Source: CAD feature listing. Evaluate the final solid. Frame: model axes, mm. A direction names the side the tool comes from. Round coordinates to 2 decimals unless told otherwise and drop trailing zeros. Write each loop counter-clockwise with the first axis right and the second up, starting at its lowest first coordinate (ties: lowest second). Pieces come first, ordered by that corner, then holes. Notation, with made-up numbers: M 32.5,66.25 L 74.5,66.25 A10 ccw 74.5,85.25 Z; hole C 8.25,67.5 d1. An arc over 180 degrees is marked long. Answer in a Markdown table with one row per item.
from build123d import *

# Parameters (mm, degrees)
SKETCH3_R          = 14.674629281
CUT_EXTRUDE1_DEPTH = 6.35
SKETCH4_W          = 6.858
SKETCH4_H          = 15.764878236
CUT_EXTRUDE2_DEPTH = 50.8
SKETCH7_W          = 3.175
SKETCH7_H          = 17.78
FINGERGRIP_DEPTH   = 1.651
GRIPS_START        = -20.955
GRIPS_DEPTH        = 17.78


# Read off the part's stored shape, not the designer's step: grips
with BuildPart() as part:
    # Sketch1 → Revolve3 (revolve)
    with BuildSketch(Plane(origin=(0, 0, 0), x_dir=(0, 0, -1), z_dir=(1, 0, 0)), mode=Mode.PRIVATE) as revolve3_sk:
        Polygon((54.61, 12.700000001), (54.61, 10.16), (41.91, 10.16), (22.86, 13.384649532), (0, 13.384649532), (0, 16.51), (22.86, 16.51), (41.91, 12.700000001), align=None)
    revolve(revolve3_sk.sketch.rotate(Axis((0, 0, 0), (0, 0, -1)), 90), axis=Axis((0, 0, 0), (0, 0, -1)))

    # Sketch3 → Cut-Extrude1 (cut)
    with BuildSketch(Plane.XY):
        Circle(SKETCH3_R)
    extrude(amount=-CUT_EXTRUDE1_DEPTH, mode=Mode.SUBTRACT)

    # Sketch4 → Cut-Extrude2 (cut, symmetric)
    with BuildSketch(Plane(origin=(0, 0, 0), x_dir=(0, 0, -1), z_dir=(1, 0, 0))):
        with Locations((47.117, 7.882439118)):
            Rectangle(SKETCH4_W, SKETCH4_H)
    extrude(amount=CUT_EXTRUDE2_DEPTH, both=True, mode=Mode.SUBTRACT)

    # Sketch7 → fingerGrip (add)
    with BuildSketch(Plane(origin=(0, 15.875, 0), x_dir=(-1, 0, 0), z_dir=(0, 1, 0))):
        with Locations((0, -12.065)):
            Rectangle(SKETCH7_W, SKETCH7_H)
    extrude(amount=FINGERGRIP_DEPTH)

    # grips outline → grips (add)
    with BuildSketch(Plane.XY.offset(GRIPS_START)):
        with BuildLine():
            Line((1.5875, -17.526), (1.5875, -16.433500654))
            ThreePointArc((1.5875, -16.433500654), (0, -16.51), (-1.5875, -16.433500654))
            Line((-1.5875, -16.433500654), (-1.5875, -17.526))
            Line((-1.5875, -17.526), (1.5875, -17.526))
        make_face()
        with BuildLine():
            ThreePointArc((15.02557904, -6.841934999), (14.298079416, -8.255), (13.43807904, -9.591565656))
            Line((13.43807904, -9.591565656), (14.384211227, -10.137815329))
            Line((14.384211227, -10.137815329), (15.971711227, -7.388184671))
            Line((15.971711227, -7.388184671), (15.02557904, -6.841934999))
        make_face()
        with BuildLine():
            Line((-14.384211227, -10.137815329), (-13.43807904, -9.591565656))
            ThreePointArc((-13.43807904, -9.591565656), (-14.298079416, -8.255), (-15.02557904, -6.841934999))
            Line((-15.02557904, -6.841934999), (-15.971711227, -7.388184671))
            Line((-15.971711227, -7.388184671), (-14.384211227, -10.137815329))
        make_face()
        with BuildLine():
            Line((-15.971711227, 7.388184671), (-15.02557904, 6.841934999))
            ThreePointArc((-15.02557904, 6.841934999), (-14.298079416, 8.255), (-13.43807904, 9.591565656))
            Line((-13.43807904, 9.591565656), (-14.384211227, 10.137815329))
            Line((-14.384211227, 10.137815329), (-15.971711227, 7.388184671))
        make_face()
        with BuildLine():
            ThreePointArc((13.43807904, 9.591565656), (14.298079416, 8.255), (15.02557904, 6.841934999))
            Line((15.02557904, 6.841934999), (15.971711227, 7.388184671))
            Line((15.971711227, 7.388184671), (14.384211227, 10.137815329))
            Line((14.384211227, 10.137815329), (13.43807904, 9.591565656))
        make_face()
    extrude(amount=GRIPS_DEPTH)


solid = part.part
Q1. Contact query for flat-ended pins moving along their axis: pin 1 Ø6 at (y, z) = (-9, -33) entering from -X; pin 2 Ø10 at (x, y) = (-9.5, -7) entering from +Z; pin 3 Ø0.9 at (y, z) = (17, -16.5) entering from -X; pin 4 Ø3 at (y, z) = (11, -9) entering from -X. Output: stop coordinate, or through.
Solutions:
| item | result |
|---|---|
| pin 1 | stops at x = -13.33 |
| pin 2 | stops at z = 0 |
| pin 3 | stops at x = -1.59 |
| pin 4 | stops at x = -14.75 |
Q2. Material intervals for probe 1 along Y at (x, z) = (0, -13); probe 2 along Y at (x, z) = (0, -3); probe 3 along X at (y, z) = (7, -42), sorted ascending.
Solutions:
| item | result |
|---|---|
| probe 1 | y = -17.53 to -13.38, 13.38 to 17.53 |
| probe 2 | y = -16.51 to -14.67, 14.67 to 16.51 |
| probe 3 | x = -10.6 to -7.36, 7.36 to 10.6 |
Q3. Access query for faces 4 (the flat face through (14.7, 8.5, -3.175)), 5 (the flat face through (0, 11, -43.688)), 6 (the flat face through (-1.588, 17, -12)), 7 (the flat face through (1.588, -17, -12)). Directions: +Z, -Z, +X, -X, +Y, -Y. A direction counts if a zero-diameter tool reaches every point of the face in a straight line with its end or side. Return the directions, or none.
Solutions:
| item | result |
|---|---|
| face 4 | +Z, +X, +Y |
| face 5 | +X, -X, +Y |
| face 6 | +Z, -Z, -X, +Y |
| face 7 | +Z, -Z, +X, -Y |
Q4. Section B-B (z = -15.5). Return loops of the section in (x, y).
Solutions:
| item | result |
|---|---|
| outline | M -15.97,-7.39 L -14.38,-10.14 L -13.44,-9.59 A16.51 ccw -1.59,-16.43 L -1.59,-17.53 L 1.59,-17.53 L 1.59,-16.43 A16.51 ccw 13.44,-9.59 L 14.38,-10.14 L 15.97,-7.39 L 15.03,-6.84 A16.51 ccw 15.03,6.84 L 15.97,7.39 L 14.38,10.14 L 13.44,9.59 A16.51 ccw 1.59,16.43 L 1.59,17.53 L -1.59,17.53 L -1.59,16.43 A16.51 ccw -13.44,9.59 L -14.38,10.14 L -15.97,7.39 L -15.03,6.84 A16.51 ccw -15.03,-6.84 Z; hole C 0,0 d26.77 |
Q5. Pull-direction query (X, two-part tool) for faces 1 (the flat face through (6.5, -11.9, -6.35)), 2 (the flat face through (-14.7, 8.5, -20.955)), 3 (the cylindrical face through (-1.653, -12.592, -48.349)); classes: pulls with the +X half, pulls with the -X half, needs draft (parallel to the pull), parting line crosses it, or undercut.
Solutions:
| item | result |
|---|---|
| face 1 | undercut |
| face 2 | needs draft |
| face 3 | parting line crosses it |
Q6. Section A-A (x = 0). State how many separate pieces and enclosed holes the cut face has, and give its area (3 significant figures).
Solutions:
| item | result |
|---|---|
| separate pieces | 3 |
| enclosed holes | 0 |
| area | 318 mm2 |
Q7. Section C-C (z = -47.5). Return loops of the section in (x, y), and give its area (3 significant figures).
Solutions:
| item | result |
|---|---|
| outline | M -12.7,0 A12.7 ccw 12.7,0 L 10.16,0 A10.16 cw -10.16,0 Z |
| area | 91.2 mm2 |
